```python
from build123d import *

# Parameters (mm, degrees)
F0_R      = 40
F0_R_2    = 9
F1_DEPTH  = 270
F3_W      = 15
F3_H      = 20
F4_DEPTH  = 270
F5_R      = 21
F6_DEPTH  = 10
F7_R      = 21
F8_DEPTH  = 10
F11_R     = 4
F12_DEPTH = 10
F13_R     = 4
F14_DEPTH = 10


with BuildPart() as f1:
    # F0 (on Front) → F1 (new body)
    with BuildSketch(Plane.XZ):
        Circle(F0_R)
        Circle(F0_R_2, mode=Mode.SUBTRACT)
    extrude(amount=F1_DEPTH)

    # F3 (on Front) → F4 (cut, through all)
    with BuildSketch(Plane.XZ):
        with Locations((0, 47.5)):
            Rectangle(F3_W, F3_H)
        with Locations((0, -47.5)):
            Rectangle(F3_W, F3_H)
    extrude(amount=F4_DEPTH, mode=Mode.SUBTRACT)

    # F5 (on face) → F6 (cut)
    with BuildSketch(Plane.XZ.offset(270)):
        Circle(F5_R)
    extrude(amount=-F6_DEPTH, mode=Mode.SUBTRACT)

    # F7 (on face) → F8 (cut)
    with BuildSketch(Plane(origin=(0, 0, 0), x_dir=(-1, 0, 0), z_dir=(0, 1, 0))):
        Circle(F7_R)
    extrude(amount=-F8_DEPTH, mode=Mode.SUBTRACT)

    # F9 (on Right) → F10 (revolve, cut)
    with BuildSketch(Plane.YZ):
        with BuildLine():
            Line((-120.5, 37), (-118, 37))
            Line((-118, 37), (-118, 55.05133))
            Line((-118, 55.05133), (-128, 55.05133))
            Line((-128, 55.05133), (-128, 37))
            Line((-128, 37), (-125.5, 37))
            ThreePointArc((-125.5, 37), (-123, 34.5), (-120.5, 37))
        make_face()
        with BuildLine():
            Line((-144.5, 37), (-142, 37))
            Line((-142, 37), (-142, 54.067336))
            Line((-142, 54.067336), (-152, 54.067336))
            Line((-152, 54.067336), (-152, 37))
            Line((-152, 37), (-149.5, 37))
            ThreePointArc((-149.5, 37), (-147, 34.5), (-144.5, 37))
        make_face()
    revolve(axis=Axis((0, -135, 0), (0, 1, 0)), mode=Mode.SUBTRACT)

    # F11 (on face) → F12 (cut)
    with BuildSketch(Plane.XY.offset(37.5)):
        with Locations((0, -17.5)):
            Circle(F11_R)
        with Locations((0, -57.5)):
            Circle(F11_R)
        with Locations((0, -97.5)):
            Circle(F11_R)
        with Locations((0, -252.5)):
            Circle(F11_R)
        with Locations((0, -212.5)):
            Circle(F11_R)
        with Locations((0, -172.5)):
            Circle(F11_R)
    extrude(amount=-F12_DEPTH, mode=Mode.SUBTRACT)

    # F13 (on face) → F14 (cut)
    with BuildSketch(Plane(origin=(0, 0, -37.5), x_dir=(1, 0, 0), z_dir=(0, 0, -1))):
        with BuildLine():
            Line((0, 17.5), (4, 17.5))
            ThreePointArc((4, 17.5), (2.828427, 20.328427), (0, 21.5))
            Line((0, 21.5), (0, 17.5))
        make_face()
        with BuildLine():
            ThreePointArc((4, 57.5), (-2.828427, 60.328427), (0, 53.5))
            ThreePointArc((0, 53.5), (2.828427, 54.671573), (4, 57.5))
        make_face()
        with BuildLine():
            ThreePointArc((0, 21.5), (-2.828427, 14.671573), (4, 17.5))
            Line((4, 17.5), (0, 17.5))
            Line((0, 17.5), (0, 21.5))
        make_face()
        with Locations((0, 97.5)):
            Circle(F13_R)
        with BuildLine():
            Line((0, 252.5), (4, 252.5))
            ThreePointArc((4, 252.5), (-2.828427, 255.328427), (0, 248.5))
            Line((0, 248.5), (0, 252.5))
        make_face()
        with BuildLine():
            ThreePointArc((4, 212.5), (2.828427, 215.328427), (0, 216.5))
            ThreePointArc((0, 216.5), (-2.828427, 209.671573), (4, 212.5))
        make_face()
        with BuildLine():
            ThreePointArc((0, 248.5), (2.828427, 249.671573), (4, 252.5))
            Line((4, 252.5), (0, 252.5))
            Line((0, 252.5), (0, 248.5))
        make_face()
        with Locations((0, 172.5)):
            Circle(F13_R)
    extrude(amount=-F14_DEPTH, mode=Mode.SUBTRACT)


solid = f1.part
```
The listing builds one solid part. Answer for the finished solid, in the listing's coordinates (mm). A direction names the side the tool comes from. Round coordinates to 2 decimals unless told otherwise and drop trailing zeros. Order: outer loops, then holes, each group sorted by start corner. A loop starts at its lowest first (then second) coordinate and runs counter-clockwise, first axis right, second up. Notation, with made-up numbers: (14.5, -40) -> (54.5, -40) arc R6 cw to (54.5, -35) -> close; hole circle Ø10 at (60.25, 43). An arc over 180 degrees is marked (long way). Answer as CSV lines item,"result".
Q1. A cutting plane is placed at A-A on y = -160.5. Determine the outline of the cut face in (x, z), plus the area to 3 significant figures.
Computed values:
outline,"(-7.5, -39.29) -> (-7.5, -37.5) -> (7.5, -37.5) -> (7.5, -39.29) arc R40 ccw to (7.5, 39.29) -> (7.5, 37.5) -> (-7.5, 37.5) -> (-7.5, 39.29) arc R40 ccw to start; hole circle Ø18 at (0, 0)"
area,"4,700 mm^2"
Q2. Consider line 1 (Y direction, x = -27, z = 29); line 2 (X direction, y = -107, z = 0); line 3 (Z direction, x = 0, y = -265.75). Determine where each line is inside the solid, lowest interval first. Write a range as from..to.
Computed values:
line 1,"y = -270..-152, -142..-128, -118..0"
line 2,"x = -40..-9, 9..40"
line 3,"z = -37.5..-21, 21..37.5"
Q3. A cutting plane is placed at B-B on z = -30.5. Give the number of separate pieces and of enclosed holes in the cut face, plus the area to 3 significant figures.
Computed values:
separate pieces,"1"
enclosed holes,"6"
area,"13,400 mm^2"
Q4. For a pull along Y with two mould halves and no side action, classify faces 6 (the flat face through (-5, -58, 37.5)), 7 (the cylindrical face through (-0.521, -13.534, 32.57)) as +Y half, -Y half, draft (parallel to the pull), parting line (faces both ways), or undercut.
Computed values:
face 6,"draft"
face 7,"undercut"
Q5. Which of the six approach directions +Z, -Z, +X, -X, +Y, -Y give full straight-line access (tool end or side, diameter ignored) to faces 1 (the flat face through (-5, -58, -37.5)), 2 (the flat face through (0, -172, 27.5)), 3 (the flat face through (0, -213, -27.5)), 4 (the flat face through (0, -135, 37.5)), 5 (the cylindrical face through (-36.12, -119.23, -8.02))?
Computed values:
face 1,"-Z, +Y, -Y"
face 2,"+Z"
face 3,"-Z"
face 4,"+Z, +Y, -Y"
face 5,"none"
Q6. Given pin 1 (4 mm diameter, centred on x = 1.5, y = -171.5, fed in from +Z); pin 2 (12.5 mm diameter, centred on x = 0.5, z = -7, fed in from -Y); pin 3 (10.5 mm diameter, centred on x = 0, y = -172.5, fed in from -Z), each flat-ended and moving along its own axis, determine where each tip first touches the part or whether it passes through.
Computed values:
pin 1,"stops at z = 27.5"
pin 2,"stops at y = -260"
pin 3,"stops at z = -37.5"
